from build123d import *

# Parameters (mm, degrees)
SKETCH1_R           = 67
SKETCH1_R_2         = 58
SKETCH1_W           = 40.5
SKETCH1_H           = 40.5
BOSS_EXTRUDE6_DEPTH = 325
FILLET4_R           = 5


with BuildPart() as part:
    # Sketch1 → Boss-Extrude6 (new body)
    # profile 1 of 3: a face of its own
    with BuildSketch(Plane.XY):
        Circle(SKETCH1_R)
        Circle(SKETCH1_R_2, mode=Mode.SUBTRACT)
    # profile 2 of 3: a face of its own
    with BuildSketch(Plane.XY):
        with Locations((-78.75, 0)):
            Rectangle(SKETCH1_W, SKETCH1_H)
        Polygon((-68.5, -1.08327383), (-68.5, 10.25), (-89, 10.25), (-89, -10.25), (-68.5, -10.25), align=None, mode=Mode.SUBTRACT)
    # profile 3 of 3: a face of its own
    with BuildSketch(Plane.XY):
        with Locations((78.75, 0)):
            Rectangle(SKETCH1_W, SKETCH1_H)
        Polygon((68.5, 10.25), (89, 10.25), (89, -10.25), (68.5, -10.25), (68.5, -1.08327383), align=None, mode=Mode.SUBTRACT)
    extrude(amount=BOSS_EXTRUDE6_DEPTH)

    # Fillet4
    fillet4_edges = [part.edges().sort_by_distance(p)[0] for p in [
        (0, -67, 0),
        (0, -67, 325),
        (0, 67, 0),
        (99, 20.25, 162.5),
        (99, -20.25, 162.5),
        (-99, -20.25, 162.5),
        (-99, 20.25, 162.5),
        (0, 67, 325),
    ]]
    fillet(fillet4_edges, radius=FILLET4_R)


solid = part.part
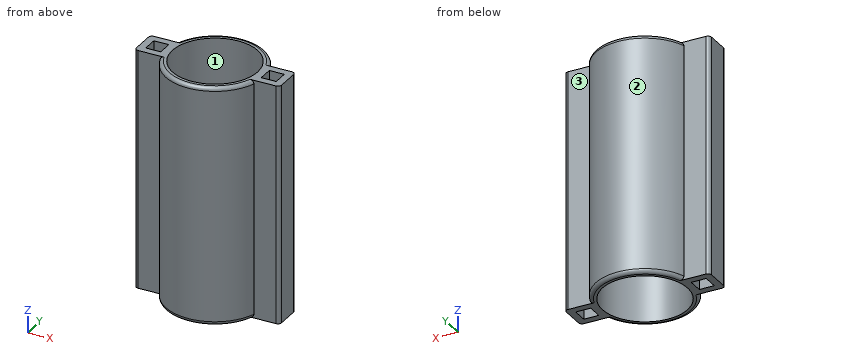
CAD build for the part. Positions are in the model's coordinates, mm. Face numbers are marked on the shaded views. Round coordinates to 2 decimals unless told otherwise and drop trailing zeros. Write each loop counter-clockwise with the first axis right and the second up, starting at its lowest first coordinate (ties: lowest second). Pieces come first, ordered by that corner, then holes.
(1) Slice it at A-A, the plane y = 0. Write the cut outline in (x, z), and give its area (3 significant figures).
(2) Mould opens along X. For the marked faces 1, 2 and 3 say: pulls with the +X half, pulls with the -X half, needs draft (parallel to the pull), parting line crosses it, or undercut.
(3) Slice it at B-B, the plane x = 0. Write the cut outline in (y, z).
(4) Drop flat-ended pins along their axis: P1, Ø3, axis at x = 67.5, z = 38, coming from the +Y side; P2, Ø8, axis at y = -42.5, z = 234.5, coming from the +X side; P3, Ø8, axis at y = -49, z = 172, coming from the +X side; P4, Ø8, axis at x = -48.5, y = -12.5, coming from the -Z side. Give the stop position or say it passes through.
(5) Slice it at C-C, the plane z = 54. Write the cut outline in (x, y).
(6) Probe line 1 along X through (y, z) = (-1, 177.5); line 2 along Y through (x, z) = (0, 257); line 3 along X through (y, z) = (-3.5, 169.5). List the from-to ranges inside material, lowest first.
From the geometry:
1. outline: (-99, 0) - (-89, 0) - (-89, 325) - (-99, 325) - close; (-68.5, 0) - (-58, 0) - (-58, 325) - (-68.5, 325) - close; (58, 0) - (68.5, 0) - (68.5, 325) - (58, 325) - close; (89, 0) - (99, 0) - (99, 325) - (89, 325) - close
1. area: 13,300 mm2
2. face 1: undercut
2. face 2: parting line crosses it
2. face 3: needs draft
3. outline: (-67, 5) arc R5 ccw to (-62, 0) - (-58, 0) - (-58, 325) - (-62, 325) arc R5 ccw to (-67, 320) - close; (58, 0) - (62, 0) arc R5 ccw to (67, 5) - (67, 320) arc R5 ccw to (62, 325) - (58, 325) - close
4. P1: stops at y = 20.25
4. P2: stops at x = 54.83
4. P3: stops at x = 49.64
4. P4: passes through
5. outline: (-99, -15.25) arc R5 ccw to (-94, -20.25) - (-63.87, -20.25) arc R67 ccw to (63.87, -20.25) - (94, -20.25) arc R5 ccw to (99, -15.25) - (99, 15.25) arc R5 ccw to (94, 20.25) - (63.87, 20.25) arc R67 ccw to (-63.87, 20.25) - (-94, 20.25) arc R5 ccw to (-99, 15.25) - close; hole (-89, -10.25) - (-68.5, -10.25) - (-68.5, 10.25) - (-89, 10.25) - close; hole circle Ø116 at (0, 0); hole (68.5, -10.25) - (89, -10.25) - (89, 10.25) - (68.5, 10.25) - close
6. line 1: x = -99 to -89, -68.5 to -57.99, 57.99 to 68.5, 89 to 99
6. line 2: y = -67 to -58, 58 to 67
6. line 3: x = -99 to -89, -68.5 to -57.89, 57.89 to 68.5, 89 to 99
